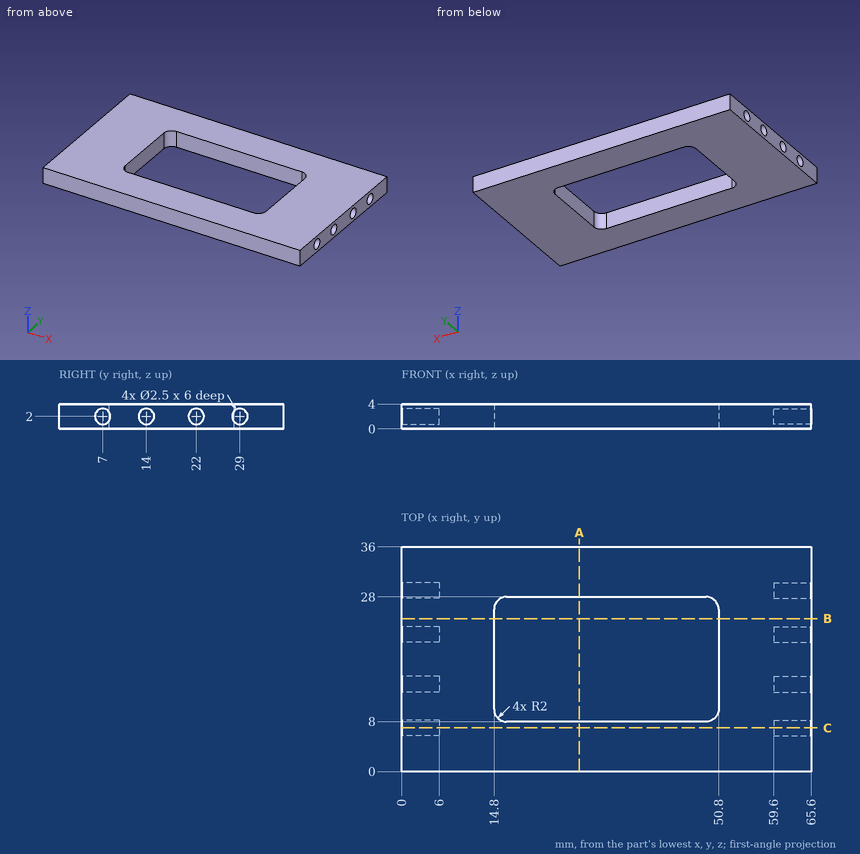
For this review, use the dimensioned drawing (mm, ordinates from the lowest corner) and the shaded views. Round coordinates to 2 decimals unless told otherwise and drop trailing zeros. Order: outer loops, then holes, each group sorted by start corner. A loop starts at its lowest first (then second) coordinate and runs counter-clockwise, first axis right, second up. Notation, with made-up numbers: M 19.5,49.25 L 42.5,49.25 A32 cw 42.5,77.25 Z; hole C 67,72.5 d4. An arc over 180 degrees is marked long. Use a Markdown table: item, result. Add a question column.
Item 1: Add section B-B, the plane y = 24.5. Give the boundary of the cut face in (x, z).
Item 2: Add section A-A, the plane x = 28.5. Give the boundary of the cut face in (y, z), then the cut area to 3 significant figures.
Item 3: To check wall thickness, follow line 1 along Y through (x, z) = (64.05, 2); line 2 along Y through (x, z) = (47, 0.8); line 3 along Y through (x, z) = (61, 2.5). State the ranges of each line that lie inside material, in increasing order.
Item 4: Insertion check: pin 1 (1.5 mm diameter, centred on y = 14, z = 2, fed in from +X); pin 2 (1 mm diameter, centred on x = 54.5, y = 19.5, fed in from -Z); pin 3 (2 mm diameter, centred on y = 29, z = 2, fed in from -X). Each pin has a flat end and moves straight along its axis. Give the tip position at first contact, or say it passes through.
Item 5: Add section C-C, the plane y = 7. Give the boundary of the cut face in (x, z).
Geometry results:
| question | item | result |
|---|---|---|
| 1 | outline | M 0,0 L 14.8,0 L 14.8,4 L 0,4 Z; M 50.8,0 L 65.6,0 L 65.6,4 L 50.8,4 Z |
| 2 | outline | M 0,0 L 8,0 L 8,4 L 0,4 Z; M 28,0 L 36,0 L 36,4 L 28,4 Z |
| 2 | area | 64.0 mm² |
| 3 | line 1 | y = 0 to 5.75, 8.25 to 12.75, 15.25 to 20.75, 23.25 to 27.75, 30.25 to 36 |
| 3 | line 2 | y = 0 to 8, 28 to 36 |
| 3 | line 3 | y = 0 to 5.85, 8.15 to 12.85, 15.15 to 20.85, 23.15 to 27.85, 30.15 to 36 |
| 4 | pin 1 | stops at x = 59.6 |
| 4 | pin 2 | stops at z = 0 |
| 4 | pin 3 | stops at x = 6 |
| 5 | outline | M 0,0 L 65.6,0 L 65.6,0.75 L 59.6,0.75 L 59.6,3.25 L 65.6,3.25 L 65.6,4 L 0,4 L 0,3.25 L 6,3.25 L 6,0.75 L 0,0.75 Z |
